Geometry check sheet. Reference: drawing and pictorial views, mm from the part's lowest x, y, z. Round coordinates to 2 decimals unless told otherwise and drop trailing zeros. Write each loop counter-clockwise with the first axis right and the second up, starting at its lowest first coordinate (ties: lowest second). Pieces come first, ordered by that corner, then holes. Notation, with made-up numbers: (32, -11) - (74, -11) arc R16 cw to (74, -1) - close; hole circle Ø9 at (-33.75, 28). An arc over 180 degrees is marked (long way). Return JSON: item names as keys, results as strings.
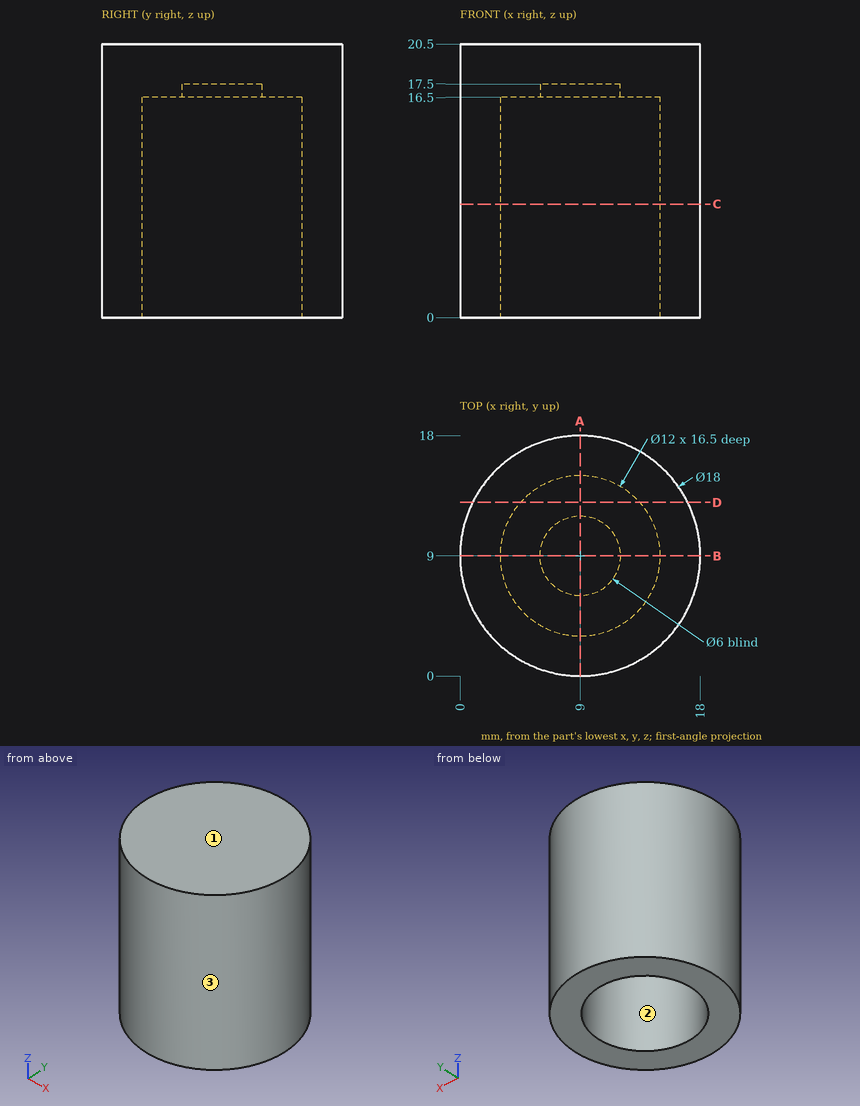
(1) Material ranges on line 1 along Y through (x, z) = (9, 17.05); line 2 along Y through (x, z) = (9, 5.75); line 3 along Z through (x, y) = (13.25, 8.25), recorded low to high. Write a range as [from, to].
Response values:
{"line 1": "y = [0, 6], [12, 18]", "line 2": "y = [0, 3], [15, 18]", "line 3": "z = [16.5, 20.5]"}
(2) Gauge pin test, flat ends, axial feed: pin 1 (3.5 mm diameter, centred on x = 7.5, y = 10.5, fed in from -Z); pin 2 (3 mm diameter, centred on y = 11.5, z = 13.5, fed in from +X); pin 3 (3 mm diameter, centred on x = 7, z = 12.5, fed in from +Y). Record the tip position at first contact, or that the pin passes through.
Response values:
{"pin 1": "stops at z = 16.5", "pin 2": "stops at x = 17.94", "pin 3": "stops at y = 17.99"}
(3) Section check C-C, the plane z = 8.5. Enter the section's corners in (x, y).
Response values:
{"outline": "circle Ø18 at (9, 9); hole circle Ø12 at (9, 9)"}
(4) Release check for a two-part mould opening along X. For the marked faces 1, 2 and 3 record: pulls with the +X half, pulls with the -X half, needs draft (parallel to the pull), parting line crosses it, or undercut.
Response values:
{"face 1": "needs draft", "face 2": "undercut", "face 3": "parting line crosses it"}
(5) Section check D-D, the plane y = 13. Enter the section's corners in (x, z), plus the area to 3 significant figures.
Response values:
{"outline": "(0.94, 0) - (4.53, 0) - (4.53, 16.5) - (13.47, 16.5) - (13.47, 0) - (17.06, 0) - (17.06, 20.5) - (0.94, 20.5) - close", "area": "183 mm^2"}
(6) Section check A-A, the plane x = 9. Enter the section's corners in (y, z).
Response values:
{"outline": "(0, 0) - (3, 0) - (3, 16.5) - (6, 16.5) - (6, 17.5) - (12, 17.5) - (12, 16.5) - (15, 16.5) - (15, 0) - (18, 0) - (18, 20.5) - (0, 20.5) - close"}
